from build123d import *

# Parameters (mm, degrees)
SKETCH_1_W               = 40
SKETCH_1_H               = 75
EXTRUDE_1_DEPTH          = 21
FILLET_1_R               = 20
CHAMFER_1_SIZE           = 10
EXTRUDE_2_DEPTH          = 700
SKETCH_3_R               = 19
EXTRUDE_4_DEPTH          = 74
SKETCH_4_W               = 17
SKETCH_4_H               = 17
EXTRUDE_5_DEPTH          = 19
SKETCH_5_R               = 3
CUT_EXTRUDE_1_DEPTH      = 19
SKETCH_6_R               = 10
EXTRUDE_6_DEPTH          = 16.5
SKETCH_7_R               = 20
EXTRUDE_7_DEPTH          = 20
SKETCH_8_W               = 50
SKETCH_8_H               = 57.5
EXTRUDE_8_DEPTH          = 2
SKETCH_9_W               = 2
SKETCH_9_H               = 57.5
EXTRUDE_9_DEPTH          = 24.5
SKETCH_10_W              = 2
SKETCH_10_H              = 42
EXTRUDE_10_DEPTH         = 24.5
SKETCH_11_R              = 1.5
CUT_EXTRUDE_2_DEPTH      = 10
SKETCH_12_R              = 1.5
CUT_EXTRUDE_3_DEPTH      = 10
SKETCH_13_R              = 1.5
CUT_EXTRUDE_4_DEPTH      = 10
CUT_EXTRUDE_5_DEPTH      = 767.033982601
CUT_EXTRUDE_5_DEPTH_BACK = 767.033982601
SKETCH_14_W              = 811.309857384
SKETCH_14_H              = 283.720617643


with BuildPart() as part:
    # 草图1 → 凸台-拉伸1 (new body)
    with BuildSketch(Plane.XY):
        Rectangle(SKETCH_1_W, SKETCH_1_H)
    extrude(amount=EXTRUDE_1_DEPTH)

    # 圆角1
    fillet_1_edges = [part.edges().sort_by_distance(p)[0] for p in [
        (-20, 37.5, 10.5),
        (20, 37.5, 10.5),
    ]]
    fillet(fillet_1_edges, radius=FILLET_1_R - 0.0001)  # a hair under: the kernel refuses the full size

    # 倒角1
    chamfer_1_edges = [part.edges().sort_by_distance(p)[0] for p in [
        (20, -37.5, 10.5),
        (-20, -37.5, 10.5),
    ]]
    chamfer(chamfer_1_edges, length=CHAMFER_1_SIZE)

    # 草图2 → 凸台-拉伸2 (add)
    with BuildSketch(Plane(origin=(0, 0, 0), x_dir=(-1, 0, 0), z_dir=(0, 0, -1))):
        with BuildLine():
            Line((-10, -37.5), (10, -37.5))
            Line((10, -37.5), (14.449874371, -21.525062814))
            ThreePointArc((14.449874371, -21.525062814), (0, -2.5), (-14.449874371, -21.525062814))
            Line((-14.449874371, -21.525062814), (-10, -37.5))
        make_face()
    extrude(amount=EXTRUDE_2_DEPTH)

    # 草图3 → 凸台-拉伸4 (add)
    with BuildSketch(Plane(origin=(0, 0, 0), x_dir=(-1, 0, 0), z_dir=(0, 0, -1))):
        with Locations(Location((0, 17.5, 0), (0, 0, 180))):
            Circle(SKETCH_3_R)
    extrude(amount=EXTRUDE_4_DEPTH)

    # 草图4 → 凸台-拉伸5 (add)
    with BuildSketch(Plane.XY.offset(21)):
        with Locations((0, -16.5)):
            Rectangle(SKETCH_4_W, SKETCH_4_H)
    extrude(amount=EXTRUDE_5_DEPTH)

    # 草图5 → 切除-拉伸1 (cut)
    with BuildSketch(Plane.ZY.offset(8.5)):
        with Locations(Location((31.5, -16.5, 0), (0, 0, 270))):
            Circle(SKETCH_5_R)
    extrude(amount=-CUT_EXTRUDE_1_DEPTH, mode=Mode.SUBTRACT)

    # 草图6 → 凸台-拉伸6 (add)
    with BuildSketch(Plane(origin=(0, 0, -700), x_dir=(-1, 0, 0), z_dir=(0, 0, -1))):
        with Locations((0, -17.5)):
            Circle(SKETCH_6_R)
    extrude(amount=EXTRUDE_6_DEPTH)

    # 草图7 → 凸台-拉伸7 (add)
    with BuildSketch(Plane(origin=(0, 0, -716.5), x_dir=(-1, 0, 0), z_dir=(0, 0, -1))):
        with Locations((0, -17.5)):
            Circle(SKETCH_7_R)
    extrude(amount=EXTRUDE_7_DEPTH)

    # 草图8 → 凸台-拉伸8 (add)
    with BuildSketch(Plane(origin=(0, 0, -736.5), x_dir=(-1, 0, 0), z_dir=(0, 0, -1))):
        with Locations((0, -17.5)):
            Rectangle(SKETCH_8_W, SKETCH_8_H)
    extrude(amount=EXTRUDE_8_DEPTH)

    # 草图9 → 凸台-拉伸9 (add)
    with BuildSketch(Plane(origin=(0, 0, -738.5), x_dir=(-1, 0, 0), z_dir=(0, 0, -1))):
        with Locations((24, -17.5)):
            Rectangle(SKETCH_9_W, SKETCH_9_H)
    extrude(amount=EXTRUDE_9_DEPTH)

    # 草图10 → 凸台-拉伸10 (add)
    with BuildSketch(Plane(origin=(0, 0, -738.5), x_dir=(-1, 0, 0), z_dir=(0, 0, -1))):
        with Locations((-24, -17.25)):
            Rectangle(SKETCH_10_W, SKETCH_10_H)
    extrude(amount=EXTRUDE_10_DEPTH)

    # 草图11 → 切除-拉伸2 (cut)
    with BuildSketch(Plane.ZY.offset(25)):
        with Locations(Location((-757, 7.25, 0), (0, 0, 270))):
            Circle(SKETCH_11_R)
        with Locations(Location((-747.1, 7.25, 0), (0, 0, 270))):
            Circle(SKETCH_11_R)
        with Locations(Location((-747.1, -41.75, 0), (0, 0, 270))):
            Circle(SKETCH_11_R)
        with Locations(Location((-757, -41.75, 0), (0, 0, 270))):
            Circle(SKETCH_11_R)
    extrude(amount=-CUT_EXTRUDE_2_DEPTH, mode=Mode.SUBTRACT)

    # 草图12 → 切除-拉伸3 (cut)
    with BuildSketch(Plane.ZY.offset(25)):
        with Locations(Location((-752.05, -31.25, 0), (0, 0, 270))):
            Circle(SKETCH_12_R)
    extrude(amount=-CUT_EXTRUDE_3_DEPTH, mode=Mode.SUBTRACT)

    # 草图13 → 切除-拉伸4 (cut)
    with BuildSketch(Plane(origin=(25, 0, 0), x_dir=(0, 0, -1), z_dir=(1, 0, 0))):
        with Locations(Location((751.5, -7.25, 0), (0, 0, 90))):
            Circle(SKETCH_13_R)
        with Locations(Location((751.5, -31.25, 0), (0, 0, 90))):
            Circle(SKETCH_13_R)
    extrude(amount=-CUT_EXTRUDE_4_DEPTH, mode=Mode.SUBTRACT)

    # 草图14 → 切除-拉伸5 (cut, two sides: drawn at the far end of the back side and taken through both)
    with BuildSketch(Plane.ZY.offset(25).offset(-CUT_EXTRUDE_5_DEPTH_BACK)):
        with Locations((-330.845071308, -36.311792758)):
            Rectangle(SKETCH_14_W, SKETCH_14_H)
    extrude(amount=CUT_EXTRUDE_5_DEPTH + CUT_EXTRUDE_5_DEPTH_BACK, mode=Mode.SUBTRACT)


solid = part.part
Geometry check sheet. Reference: the model listing, model coordinates, mm. A direction names the side the tool comes from. Round coordinates to 2 decimals unless told otherwise and drop trailing zeros. Order: outer loops, then holes, each group sorted by start corner. A loop starts at its lowest first (then second) coordinate and runs counter-clockwise, first axis right, second up. Notation, with made-up numbers: M 4.5,-22.75 L 45.5,-22.75 A31 cw 45.5,12.25 Z; hole C 85,61 d5. An arc over 180 degrees is marked long. Write each question's results on one line, items separated by ' | '. Start each with the question number.
1. Draft check along X on faces 6 (the face through (-25, -18, -750)), 7 (the face through (1, -17, -738.5)), 8 (the face through (-7, 11.25, -738)). Enter one of: pulls with the +X half, pulls with the -X half, needs draft (parallel to the pull), parting line crosses it, or undercut.
2. Cross-section at B-B on z = -747.1. Record the boundary of the cut face in (x, y).
3. Cross-section at C-C on z = -754.5. Record the boundary of the cut face in (x, y), plus the area to 3 significant figures.
4. Set-up check for faces 1 (the face through (23, -18, -751)), 2 (the face through (24.014, -7.445, -750.013)), 3 (the face through (-24.01, -30.06, -752.96)), 4 (the face through (24, 3.75, -751)), 5 (the face through (24, -38.25, -751)): record each of +Z, -Z, +X, -X, +Y, -Y from which the full face is reachable in a straight line by a thin tool's end or side.
5. Material ranges on L1, parallel to Y at x = -24, z = -757; L2, parallel to Z at x = -24.6, y = 7.25; L3, parallel to X at y = -23.5, z = -746.75, recorded low to high. Write a range as from..to.
6. Cross-section at D-D on y = -1.5. Record the boundary of the cut face in (x, z).
7. Cross-section at A-A on y = 7.25. Record the boundary of the cut face in (x, z), plus the area to 3 significant figures.
8. Go/stop test with flat-tipped pins: P1, Ø1, axis at x = 24, z = -746, coming from the -Y side; P2, Ø0.6, axis at x = 24, z = -752, coming from the +Y side; P3, Ø3.5, axis at y = -41.75, z = -757, coming from the -X side; P4, Ø6, axis at x = 5, y = -37, coming from the -Z side. Record where each tip stops, or that it passes through.
Resolved:
1) face 6: pulls with the -X half | face 7: undercut | face 8: needs draft
2) outline: M -25,-46.25 L -23,-46.25 L -23,-43.25 L -25,-43.25 Z; M -25,-40.25 L -23,-40.25 L -23,5.75 L -25,5.75 Z; M -25,8.75 L -23,8.75 L -23,11.25 L -25,11.25 Z; M 23,-38.25 L 25,-38.25 L 25,3.75 L 23,3.75 Z
3) outline: M -25,-46.25 L -23,-46.25 L -23,11.25 L -25,11.25 Z; M 23,-38.25 L 25,-38.25 L 25,3.75 L 23,3.75 Z | area: 199 mm2
4) face 1: -Z, +Y, -Y | face 2: +X | face 3: -X | face 4: -Z, +X, +Y | face 5: -Z, +X, -Y
5) L1: -46.25..-43.25, -40.25..5.75, 8.75..11.25 | L2: -763..-758.5, -755.5..-748.6, -745.6..-736.5 | L3: -25..-23, 23..25
6) outline: M -25,-763 L -23,-763 L -23,-738.5 L 23,-738.5 L 23,-763 L 25,-763 L 25,-736.5 L -25,-736.5 Z
7) outline: M -25,-763 L -23,-763 L -23,-758.5 L -25,-758.5 Z; M -25,-755.5 L -23,-755.5 L -23,-748.6 L -25,-748.6 Z; M -25,-745.6 L -23,-745.6 L -23,-738.5 L 25,-738.5 L 25,-736.5 L -25,-736.5 Z | area: 137 mm2
8) P1: y = -38.25 | P2: y = 3.75 | P3: x = -25 | P4: z = -738.5
